```python
from build123d import *

# Parameters (mm, degrees)
SKETCH_1_R      = 6
SKETCH_1_R_2    = 3
EXTRUDE_1_DEPTH = 2
SKETCH_2_R      = 6.75
SKETCH_2_R_2    = 3
EXTRUDE_2_DEPTH = 1
CHAMFER_1_SIZE  = 0.2


with BuildPart() as part:
    # 草图1 → 凸台-拉伸1 (new body, symmetric)
    with BuildSketch(Plane.XY):
        Circle(SKETCH_1_R)
        Circle(SKETCH_1_R_2, mode=Mode.SUBTRACT)
    extrude(amount=EXTRUDE_1_DEPTH, both=True)

    # 草图2 → 凸台-拉伸2 (add)
    with BuildSketch(Plane.XY.offset(2)):
        Circle(SKETCH_2_R)
        Circle(SKETCH_2_R_2, mode=Mode.SUBTRACT)
    extrude(amount=-EXTRUDE_2_DEPTH)

    # 倒角1
    chamfer_1_edges = [part.edges().sort_by_distance(p)[0] for p in [
        (-6.75, 0, 2),
        (-6.75, 0, 1),
        (-6, 0, -2),
    ]]
    chamfer(chamfer_1_edges, length=CHAMFER_1_SIZE)


solid = part.part
```
Geometry check sheet. Reference: the model listing, model coordinates, mm. A direction names the side the tool comes from. Round coordinates to 2 decimals unless told otherwise and drop trailing zeros. Loops run counter-clockwise (first coordinate to the right, second up) from the corner with the lowest first, then second, coordinate; pieces in that order, holes last. Notation, with made-up numbers: (17, 77.5) -> (76, 77.5) arc R19 ccw to (76, 94.5) -> close; hole circle Ø2 at (-25, -35.75). An arc over 180 degrees is marked (long way). Use a Markdown table: item, result.
(1) Mould release check, pull along X, two halves, no side actions. Record for faces 1 (the cylindrical face through (-3, 0, 0)), 2 (the cylindrical face through (-1.46, -6.59, 1.5)), 3 (the flat face through (2.5, -2.5, -2)): released by +X, released by -X, zero draft, split by the parting line, or undercut.
Calculated:
| item | result |
|---|---|
| face 1 | undercut |
| face 2 | split by the parting line |
| face 3 | zero draft |
(2) Go/stop test with flat-tipped pins: P1, Ø2, axis at y = 1, z = -0.5, coming from the +X side; P2, Ø3, axis at x = -1, y = -0.5, coming from the -Z side. Record where each tip stops, or that it passes through.
Calculated:
| item | result |
|---|---|
| P1 | x = 6 |
| P2 | through |
(3) Sectioned sample at A-A (x = 0). Enter the section's corners in (y, z), then the cut area to 3 significant figures.
Calculated:
| item | result |
|---|---|
| outline | (-6.75, 1.2) -> (-6.55, 1) -> (-6, 1) -> (-6, -1.8) -> (-5.8, -2) -> (-3, -2) -> (-3, 2) -> (-6.55, 2) -> (-6.75, 1.8) -> close; (3, -2) -> (5.8, -2) -> (6, -1.8) -> (6, 1) -> (6.55, 1) -> (6.75, 1.2) -> (6.75, 1.8) -> (6.55, 2) -> (3, 2) -> close |
| area | 25.4 mm² |
(4) Scan lines: probe 1 along Y at (x, z) = (-2.75, -0.2); probe 2 along Y at (x, z) = (2.25, 1.4); probe 3 along X at (y, z) = (2.25, -0.7). Record each from-to range of solid material in increasing order.
Calculated:
| item | result |
|---|---|
| probe 1 | -5.33 to -1.2, 1.2 to 5.33 |
| probe 2 | -6.36 to -1.98, 1.98 to 6.36 |
| probe 3 | -5.56 to -1.98, 1.98 to 5.56 |
(5) Sectioned sample at C-C (z = -0.35). Enter the section's corners in (x, y), then the cut area to 3 significant figures.
Calculated:
| item | result |
|---|---|
| outline | circle Ø12 at (0, 0); hole circle Ø6 at (0, 0) |
| area | 84.8 mm² |
(6) Set-up check for faces 4 (the flat face through (3, -1, 2)), 5 (the cylindrical face through (-6, 0, 0)): record each of +Z, -Z, +X, -X, +Y, -Y from which the full face is reachable in a straight line by a thin tool's end or side.
Calculated:
| item | result |
|---|---|
| face 4 | +Z, +X, -X, +Y, -Y |
| face 5 | -Z |
